```python
from build123d import *

# Parameters (mm, degrees)
SKETCH_1_W          = 10.65
SKETCH_1_H          = 32
EXTRUDE_1_DEPTH     = 1.5
CUT_EXTRUDE_START   = -1
CUT_EXTRUDE_1_DEPTH = 8.5
SKETCH_4_W          = 0.9
SKETCH_4_H          = 20
EXTRUDE_2_DEPTH     = 0.8
CUT_EXTRUDE_2_DEPTH = 5.8
CUT_EXTRUDE_3_DEPTH = 0.8
EXTRUDE_3_DEPTH     = 1
SKETCH_8_W          = 10.65
SKETCH_8_H          = 32
SKETCH_8_W_2        = 10.33
SKETCH_8_H_2        = 31.68
CUT_EXTRUDE_4_DEPTH = 10


with BuildPart() as part:
    # 草图1 → 凸台-拉伸1 (new body)
    with BuildSketch(Plane(origin=(0, 0, 0), x_dir=(1, 0, 0), z_dir=(0, 1, 0))):
        with Locations((5.325, -16)):
            Rectangle(SKETCH_1_W, SKETCH_1_H)
    extrude(amount=EXTRUDE_1_DEPTH)

    # 草图3 → 切除-拉伸1 (cut)
    with BuildSketch(Plane.ZY.offset(CUT_EXTRUDE_START)):
        Polygon((22.619658117, 1.5), (29.745922722, 1.5), (22.619658117, 0.65), align=None)
    extrude(amount=-CUT_EXTRUDE_1_DEPTH, mode=Mode.SUBTRACT)

    # 草图4 → 凸台-拉伸2 (add)
    with BuildSketch(Plane(origin=(0, 1.5, 0), x_dir=(1, 0, 0), z_dir=(0, 1, 0))):
        with Locations((1.6, -11)):
            Rectangle(SKETCH_4_W, SKETCH_4_H)
        with Locations((9.05, -11)):
            Rectangle(SKETCH_4_W, SKETCH_4_H)
    extrude(amount=EXTRUDE_2_DEPTH)

    # 草图5 → 切除-拉伸2 (cut)
    with BuildSketch(Plane(origin=(0, 1.5, 0), x_dir=(1, 0, 0), z_dir=(0, 1, 0))):
        with BuildLine():
            Line((3.25, -15.60411185), (3.25, -20.495209364))
            ThreePointArc((3.25, -20.495209364), (3.367157288, -20.778052076), (3.65, -20.895209364))
            Line((3.65, -20.895209364), (6.85, -20.895209364))
            ThreePointArc((6.85, -20.895209364), (7.132842712, -20.778052076), (7.25, -20.495209364))
            Line((7.25, -20.495209364), (7.25, -17.536917794))
            ThreePointArc((7.25, -17.536917794), (7.198369033, -17.340349696), (7.056804915, -17.194526604))
            Line((7.056804915, -17.194526604), (3.856804915, -15.261720659))
            ThreePointArc((3.856804915, -15.261720659), (3.453431902, -15.255742817), (3.25, -15.60411185))
        make_face()
        with BuildLine():
            Line((3.510326299, -14.380458294), (6.436346003, -16.139397213))
            ThreePointArc((6.436346003, -16.139397213), (6.977388991, -16.14656228), (7.25, -15.679162997))
            Line((7.25, -15.679162997), (7.25, -12.569402982))
            ThreePointArc((7.25, -12.569402982), (7.029399053, -12.135517868), (6.548846383, -12.05812148))
            Line((6.548846383, -12.05812148), (3.713121915, -12.968622573))
            ThreePointArc((3.713121915, -12.968622573), (3.378076137, -13.210716019), (3.25, -13.603731812))
            Line((3.25, -13.603731812), (3.25, -13.920224078))
            ThreePointArc((3.25, -13.920224078), (3.319590865, -14.184603216), (3.510326299, -14.380458294))
        make_face()
    extrude(amount=-CUT_EXTRUDE_2_DEPTH, mode=Mode.SUBTRACT)

    # 草图6 → 切除-拉伸3 (cut)
    with BuildSketch(Plane(origin=(0, 2.3, 0), x_dir=(1, 0, 0), z_dir=(0, 1, 0))):
        Polygon((9.5, -7.744189198), (8.6, -9.370124246), (8.6, -11), (9.5, -9.374064951), align=None)
    extrude(amount=-CUT_EXTRUDE_3_DEPTH, mode=Mode.SUBTRACT)

    # 草图7 → 凸台-拉伸3 (add)
    with BuildSketch(Plane(origin=(0, -2.01927835, 0.240853616), x_dir=(1, 0, 0), z_dir=(0, 0.9929615038625476, -0.11843754407715576))):
        Polygon((2.308389857, -23.863899052), (7.814564381, -23.863899052), (5.511982308, -28.494091265), (2.308389857, -28.494091265), align=None)
    extrude(amount=EXTRUDE_3_DEPTH)

    # 草图8 → 切除-拉伸4 (cut)
    with BuildSketch(Plane(origin=(0, 1.5, 0), x_dir=(1, 0, 0), z_dir=(0, 1, 0))):
        with Locations((5.325, -16)):
            Rectangle(SKETCH_8_W, SKETCH_8_H)
        with Locations((5.325, -16)):
            Rectangle(SKETCH_8_W_2, SKETCH_8_H_2, mode=Mode.SUBTRACT)
    extrude(amount=-CUT_EXTRUDE_4_DEPTH, mode=Mode.SUBTRACT)


solid = part.part
```
Geometry check sheet. Reference: the model listing, model coordinates, mm. A direction names the side the tool comes from. Give positions to 0.01 mm unless a question says otherwise; leave off trailing zeros. Order: outer loops, then holes, each group sorted by start corner. A loop starts at its lowest first (then second) coordinate and runs counter-clockwise, first axis right, second up. Notation, with made-up numbers: (89, -11.5) - (111, -11.5) arc R29 cw to (111, 19.5) - close; hole circle Ø3 at (-31, 29). An arc over 180 degrees is marked (long way). Answer in a Markdown table with one row per item. Add a question column.
Q1. Tool access check on faces 5 (the flat face through (5, 1, 20.895)), 6 (the flat face through (2.308, 1.6, 26.2)), 7 (the flat face through (5, 1, 0.16)). Record the directions out of +Z, -Z, +X, -X, +Y, -Y that give a thin tool (end or side, any length) a straight path to the whole face; none if there is none.
Q2. Cross-section at A-A, the plane x = 5. Enter the section's corners in (y, z).
Q3. Cross-section at D-D, the plane z = 11.5. Enter the section's corners in (x, y), then the cut area to 3 significant figures.
Q4. Gauge pin test, flat ends, axial feed: pin 1 (4 mm diameter, centred on x = 6, z = 11, fed in from +Y); pin 2 (0.9 mm diameter, centred on y = 2, z = 14, fed in from -X); pin 3 (0.5 mm diameter, centred on x = 1.5, z = 9, fed in from +Y); pin 4 (5 mm diameter, centred on x = 7.5, z = 19, fed in from -Y). Record the tip position at first contact, or that the pin passes through.
Q5. Cross-section at C-C, the plane z = 27.5. Enter the section's corners in (x, y).
Q6. Mould release check, pull along X, two halves, no side actions. Record for faces 1 (the flat face through (0.16, 1, 16)), 2 (the flat face through (9, 2.3, 5)), 3 (the flat face through (5.02, 1.3, 23.88)), 4 (the flat face through (9.056, 1.906, 8.546)): pulls with the +X half, pulls with the -X half, needs draft (parallel to the pull), parting line crosses it, or undercut.
Q7. Cross-section at B-B, the plane y = 0.3. Enter the section's corners in (x, z), then the cut area to 3 significant figures.
Q8. Material ranges on probe 1 along X at (y, z) = (2.15, 4); probe 2 along Z at (x, y) = (5.5, 0.1); probe 3 along Z at (x, y) = (6, 0.4), recorded low to high. Write a range as from..to.
Check values:
| question | item | result |
|---|---|---|
| 1 | face 5 | +Y, -Y |
| 1 | face 6 | +Y |
| 1 | face 7 | -Z, +X, -X, +Y, -Y |
| 2 | outline | (0, 0.16) - (1.5, 0.16) - (1.5, 12.56) - (0, 12.56) - close; (0, 15.28) - (1.5, 15.28) - (1.5, 15.95) - (0, 15.95) - close; (0, 20.9) - (1.5, 20.9) - (1.5, 22.62) - (0.65, 22.62) - (0.81, 23.94) - (1.8, 23.82) - (2.35, 28.42) - (1.36, 28.53) - (1.5, 29.75) - (1.5, 31.84) - (0, 31.84) - close |
| 3 | outline | (0.16, 0) - (10.49, 0) - (10.49, 1.5) - (9.5, 1.5) - (9.5, 2.3) - (8.6, 2.3) - (8.6, 1.5) - (2.05, 1.5) - (2.05, 2.3) - (1.15, 2.3) - (1.15, 1.5) - (0.16, 1.5) - close |
| 3 | area | 16.9 mm^2 |
| 4 | pin 1 | stops at y = 1.5 |
| 4 | pin 2 | stops at x = 1.15 |
| 4 | pin 3 | stops at y = 2.3 |
| 4 | pin 4 | stops at y = 0 |
| 5 | outline | (0.16, 0) - (10.49, 0) - (10.49, 1.5) - (9.5, 1.5) - (9.5, 1.23) - (6.03, 1.23) - (5.97, 2.24) - (2.31, 2.24) - (2.31, 1.23) - (1, 1.23) - (1, 1.5) - (0.16, 1.5) - close |
| 6 | face 1 | pulls with the -X half |
| 6 | face 2 | needs draft |
| 6 | face 3 | undercut |
| 6 | face 4 | pulls with the +X half |
| 7 | outline | (0.16, 0.16) - (10.49, 0.16) - (10.49, 31.84) - (0.16, 31.84) - close; hole (3.25, 13.6) arc R0.67 ccw to (3.71, 12.97) - (6.55, 12.06) arc R0.54 ccw to (7.25, 12.57) - (7.25, 15.68) arc R0.54 ccw to (6.44, 16.14) - (3.51, 14.38) arc R0.54 ccw to (3.25, 13.92) - close; hole (3.25, 15.6) arc R0.4 ccw to (3.86, 15.26) - (7.06, 17.19) arc R0.4 ccw to (7.25, 17.54) - (7.25, 20.5) arc R0.4 ccw to (6.85, 20.9) - (3.65, 20.9) arc R0.4 ccw to (3.25, 20.5) - close |
| 7 | area | 297 mm^2 |
| 8 | probe 1 | x = 1.15..2.05, 8.6..9.5 |
| 8 | probe 2 | z = 0.16..12.39, 15.58..16.25, 20.9..31.84 |
| 8 | probe 3 | z = 0.16..12.23, 15.88..16.56, 20.9..31.84 |
